Can you work these out from the model? Positions are in its coordinate system, mm. A direction names the side the tool comes from. Give positions to 0.01 mm unless a question says otherwise; leave off trailing zeros. Order: outer loops, then holes, each group sorted by start corner. A loop starts at its lowest first (then second) coordinate and runs counter-clockwise, first axis right, second up. Notation, with made-up numbers: M 28.25,10.25 L 70.25,10.25 A22 cw 70.25,24.25 Z; hole C -13.75,57.5 d4. An arc over 180 degrees is marked long. Answer as a JSON object with one key per item and string values.
```python
from build123d import *

# Parameters (mm, degrees)
BOSS_EXTRUDE1_DEPTH     = 6.35
CAVITY1_START           = -18.343561252
CAVITY1_OUTLINE_R       = 12.7
CAVITY1_DEPTH           = 21.704189785
CUT_EXTRUDE1_REACH      = 334.451
CUT_EXTRUDE1_END_RADIUS = 12.7
SKETCH3_W               = 25.4
SKETCH3_H               = 12.7


# Read off the part's stored shape, not the designer's step: Cavity1
with BuildPart() as part:
    # Sketch1 → Boss-Extrude1 (new, symmetric)
    with BuildSketch(Plane(origin=(0, 0, 0), x_dir=(1, 0, 0), z_dir=(0, 1, 0))):
        Polygon((-215.9, -139.7), (215.9, -139.7), (215.9, -63.5), (241.3, -63.5), (241.3, 12.7), (215.9, 12.7), (215.9, 88.9), (-215.9, 88.9), (-215.9, 12.7), (-241.3, 12.7), (-241.3, -63.5), (-215.9, -63.5), align=None)
    extrude(amount=BOSS_EXTRUDE1_DEPTH, both=True)

    # Cavity1 outline → Cavity1 (cut)
    with BuildSketch(Plane(origin=(0, 0, 0), x_dir=(1, 0, 0), z_dir=(0, 0.9501228611580823, 0.3118758546357501)).offset(CAVITY1_START)):
        with Locations((-50.8, 22.822585801)):
            Circle(CAVITY1_OUTLINE_R)
    extrude(amount=CAVITY1_DEPTH, mode=Mode.SUBTRACT)

    # Cut-Extrude1: up to this cylinder (the profile starts outside it)
    cut_extrude1_end = Plane(origin=(-50.8, -19.225068271, -30.3312567), z_dir=(0, 0.9501228611580824, 0.3118758546357496)) * Cylinder(CUT_EXTRUDE1_END_RADIUS, 695.302, mode=Mode.PRIVATE)
    # Sketch3 → Cut-Extrude1 (cut, up to the surface)
    with BuildSketch(Plane(origin=(0, 0, -88.9), x_dir=(-1, 0, 0), z_dir=(0, 0, -1)), mode=Mode.PRIVATE) as cut_extrude1_sk1:
        with Locations((50.8, 0)):
            Rectangle(SKETCH3_W, SKETCH3_H)
    cut_extrude1_tool1 = extrude(cut_extrude1_sk1.sketch, amount=-CUT_EXTRUDE1_REACH, mode=Mode.PRIVATE) - cut_extrude1_end
    add(cut_extrude1_tool1.solids().sort_by_distance((-50.8, 0, -88.9))[0], mode=Mode.SUBTRACT)


solid = part.part
```
1) I'm going to push flat-ended pins straight in: pin 1 Ø6.5 at (x, y) = (-224, 2) entering from -Z; pin 2 Ø4 at (y, z) = (-2, -33) entering from +X. Where does each tip first touch, or does it pass through?
Results found:
{"pin 1": "stops at z = -12.7", "pin 2": "stops at x = 215.9"}
2) I want a section at B-B on z = 68.5. Write out the boundary of the cut face in (x, y).
Results found:
{"outline": "M -215.9,-6.35 L 215.9,-6.35 L 215.9,6.35 L -215.9,6.35 Z"}
3) I need wall thicknesses on L1, parallel to X at y = 2.75, z = -65; L2, parallel to X at y = -1.75, z = 81; L3, parallel to Z at x = -51.5, y = -3.5. Which ranges of each line are inside material? Lowest first, please.
Results found:
{"L1": "x = -215.9 to -63.5, -38.1 to 215.9", "L2": "x = -215.9 to 215.9", "L3": "z = -11.82 to 139.7"}
4) Thinking about a two-plate mould opening in X: for faces 4 (the face through (-63.5, 0, -56)), 5 (the face through (-215.9, 0, -51)), 6 (the face through (215.9, 0, -50)), 7 (the face through (-228, 0, -12.7)), which applies, pulls with the +X half, pulls with the -X half, needs draft (parallel to the pull), parting line crosses it, or undercut?
Results found:
{"face 4": "undercut", "face 5": "pulls with the -X half", "face 6": "pulls with the +X half", "face 7": "needs draft"}
5) I want a section at A-A on z = -48. Write out the boundary of the cut face in (x, y).
Results found:
{"outline": "M -215.9,-6.35 L -63.5,-6.35 L -63.5,6.35 L -215.9,6.35 Z; M -38.1,-6.35 L 215.9,-6.35 L 215.9,6.35 L -38.1,6.35 Z"}
6) For faces 1 (the face through (229, 0, -12.7)), 2 (the face through (-215.9, 0, 101)), 3 (the face through (228, 0, 63.5)), which set-ups out of +Z, -Z, +X, -X, +Y, -Y let a thin tool reach every point of the face, with its end or its side?
Results found:
{"face 1": "-Z, +X, +Y, -Y", "face 2": "+Z, -X, +Y, -Y", "face 3": "+Z, +X, +Y, -Y"}
